Model file for the job. Use its own axes, mm. Face numbers are marked on the shaded views. A direction names the side the tool comes from. Give positions to 0.01 mm unless a question says otherwise; leave off trailing zeros. Order: outer loops, then holes, each group sorted by start corner. A loop starts at its lowest first (then second) coordinate and runs counter-clockwise, first axis right, second up. Notation, with made-up numbers: M 12,60 L 41,60 A17 cw 41,88 Z; hole C 50,67.25 d6. An arc over 180 degrees is marked long. Return JSON: item names as keys, results as strings. Group by question number.
1. Slice it at D-D on z = 3.5. List the corners of the cut face in (x, y) (3 decimals), then the cut area to 3 significant figures.
2. Slice it at C-C on y = 0.25. List the corners of the cut face in (x, z) (3 decimals).
3. Wall check: probe 1 along Y at (x, z) = (2, -5); probe 2 along X at (y, z) = (10, 6.25) (3 decimals); probe 3 along Z at (x, y) = (-0.25, 3.75). Give the ranges that are in metal, low to high. Write a range as [from, to].
4. Slice it at A-A on z = 1. List the corners of the cut face in (x, y) (3 decimals).
5. Two-plate mould, pull along X, no slides. Class the marked faces 1, 2 and 3: released by +X, released by -X, zero draft, split by the parting line, or undercut.
6. Pin check, flat tips, straight feed: pin 1 (0.9 mm diameter, centred on x = 0.5, z = -5, fed in from +Y); pin 2 (0.6 mm diameter, centred on x = -1.5, z = 3.5, fed in from -Y); pin 3 (1.3 mm diameter, centred on x = -0.5, z = 6, fed in from +Y); pin 4 (1.2 mm diameter, centred on x = 0, y = -4, fed in from -Z). Stop position of each tip, or through.
7. 3-axis set-ups, long thin cutter, end or side, ignore diameter. For the marked faces 4, 5 and 6: which of +Z, -Z, +X, -X, +Y, -Y reach the whole face in a straight line?
from build123d import *

# Parameters (mm, degrees)
SKETCH_1_W          = 9.55
SKETCH_1_H          = 17.7
EXTRUDE_1_DEPTH     = 14.5
SKETCH_2_W          = 8.05
SKETCH_2_H          = 14.2
CUT_EXTRUDE_1_DEPTH = 6.5
SKETCH_5_W          = 8.05
SKETCH_5_H          = 13.3
CUT_EXTRUDE_4_DEPTH = 2.5
FILLET_1_R          = 1.5
SKETCH_8_W          = 8.05
SKETCH_8_H          = 9
EXTRUDE_1320_DEPTH  = 1.5
FILLET_2_R          = 1.5
SKETCH_10_W         = 7.5
SKETCH_10_H         = 7.5
EXTRUDE_4_DEPTH     = 1.2
FILLET_4_R          = 0.5
SKETCH_11_W         = 1.5
SKETCH_11_H         = 1
EXTRUDE_1_2_DEPTH   = 7


with BuildPart() as part:
    # 草图1 → Extrude 1 (new body)
    with BuildSketch(Plane(origin=(0, 0, 0), x_dir=(1, 0, 0), z_dir=(0, 1, 0))):
        Rectangle(SKETCH_1_W, SKETCH_1_H)
    extrude(amount=EXTRUDE_1_DEPTH)

    # 草图2 → 切除-拉伸1 (cut)
    with BuildSketch(Plane(origin=(0, 14.5, 0), x_dir=(-1, 0, 0), z_dir=(0, 1, 0))):
        with Locations((0, 1.75)):
            Rectangle(SKETCH_2_W, SKETCH_2_H)
    extrude(amount=-CUT_EXTRUDE_1_DEPTH, mode=Mode.SUBTRACT)

    # 草图5 → 切除-拉伸4 (cut)
    with BuildSketch(Plane(origin=(0, 0, -8.85), x_dir=(-1, 0, 0), z_dir=(0, 0, -1))):
        with Locations((0, 6.65)):
            Rectangle(SKETCH_5_W, SKETCH_5_H)
    extrude(amount=-CUT_EXTRUDE_4_DEPTH, mode=Mode.SUBTRACT)

    # 圆角1
    fillet_1_edges = [part.edges().sort_by_distance(p)[0] for p in [
        (4.4, 14.5, 8.85),
        (-4.4, 14.5, 8.85),
    ]]
    fillet(fillet_1_edges, radius=FILLET_1_R)

    # 草图8 → Extrude 1320 (add)
    with BuildSketch(Plane(origin=(0, 8, 0), x_dir=(-1, 0, 0), z_dir=(0, 1, 0))):
        Rectangle(SKETCH_8_W, SKETCH_8_H)
    extrude(amount=EXTRUDE_1320_DEPTH)

    # 圆角2
    fillet_2_edges = [part.edges().sort_by_distance(p)[0] for p in [
        (0, 9.5, -4.5),
        (0, 9.5, 4.5),
    ]]
    fillet(fillet_2_edges, radius=FILLET_2_R - 0.0001)  # a hair under: the kernel refuses the full size

    # 草图10 → 拉伸4 (add)
    with BuildSketch(Plane(origin=(0, 9.5, 0), x_dir=(-1, 0, 0), z_dir=(0, 1, 0))):
        Rectangle(SKETCH_10_W, SKETCH_10_H)
    extrude(amount=EXTRUDE_4_DEPTH)

    # 圆角4
    fillet_4_edges = [part.edges().sort_by_distance(p)[0] for p in [
        (3.75, 10.7, 0),
        (0, 10.7, -3.75),
        (-3.75, 10.7, 0),
        (0, 10.7, 3.75),
    ]]
    fillet(fillet_4_edges, radius=FILLET_4_R)

    # 草图11 → Extrude 1 2 (add)
    with BuildSketch(Plane.XZ):
        with Locations((0, -4.15)):
            Rectangle(SKETCH_11_W, SKETCH_11_H)
    extrude(amount=EXTRUDE_1_2_DEPTH)


solid = part.part
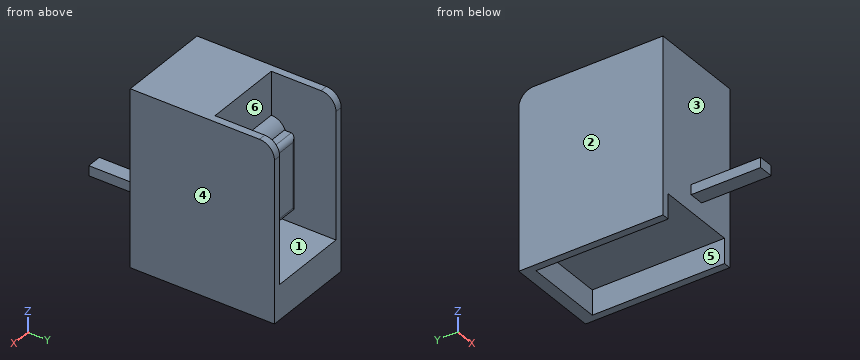
Result:
{
 "1": {"outline": "M -4.775,0 L 4.775,0 L 4.775,14.5 L 4.025,14.5 L 4.025,9.414 L -4.025,9.414 L -4.025,14.5 L -4.775,14.5 Z; M -3.75,9.5 L 3.75,9.5 L 3.75,10.2 A0.5 ccw 3.5,10.633 L -3.5,10.633 A0.5 ccw -3.75,10.2 Z", "area": "106 mm2"},
 "2": {"outline": "M -4.775,-8.85 L -4.025,-8.85 L -4.025,-6.35 L 4.025,-6.35 L 4.025,-8.85 L 4.775,-8.85 L 4.775,8.85 L -4.775,8.85 Z"},
 "3": {"probe 1": "y = [0, 8]", "probe 2": "x = [-4.775, -4.025], [4.025, 4.775]", "probe 3": "z = [-6.35, 8.85]"},
 "4": {"outline": "M -4.775,0 L 4.775,0 L 4.775,14.5 L 4.025,14.5 L 4.025,9.5 L 3.75,9.5 L 3.75,10.2 A0.5 ccw 3.25,10.7 L -3.25,10.7 A0.5 ccw -3.75,10.2 L -3.75,9.5 L -4.025,9.5 L -4.025,14.5 L -4.775,14.5 Z"},
 "5": {"face 1": "undercut", "face 2": "released by -X", "face 3": "zero draft"},
 "6": {"pin 1": "stops at y = 14.5", "pin 2": "stops at y = 0", "pin 3": "stops at y = 8", "pin 4": "stops at z = -4.65"},
 "7": {"face 4": "+Z, -Z, +X, +Y, -Y", "face 5": "-Z, -Y", "face 6": "+Z, +Y"}
}
